Source: CAD feature listing. Evaluate the final solid. Frame: model axes, mm. Face numbers are marked on the shaded views. A direction names the side the tool comes from. Round coordinates to 2 decimals unless told otherwise and drop trailing zeros. Loops run counter-clockwise (first coordinate to the right, second up) from the corner with the lowest first, then second, coordinate; pieces in that order, holes last. Notation, with made-up numbers: M 77.5,53.5 L 122.5,53.5 A33 cw 122.5,90.5 Z; hole C 18.25,71.25 d5. An arc over 180 degrees is marked long. Answer as CSV lines item,"result". Start each with the question number.
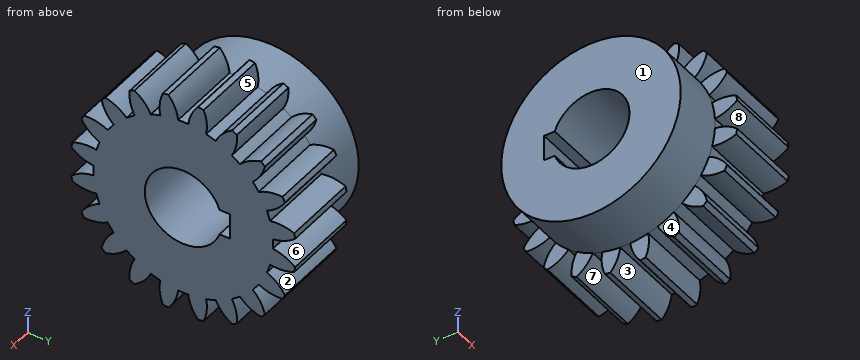
```python
from build123d import *
from build123d.topology import SkipClean

# Parameters (mm, degrees)
BASPROSKE_W      = 30
BASPROSKE_H      = 44
TOOTHCUT_DEPTH   = 70.079664157
TEETHCUTS_COUNT  = 20
TEETHCUTS_ANGLE  = 342
HUBNEARONE_START = 20.0000508
HUBNEAONESKE_R   = 34.999
HUBNEARONE_DEPTH = 20.0000508
BORSKE_R         = 15
BORE_DEPTH       = 50.0000508
KEYSKE_W         = 10
KEYSKE_H         = 18.3
KEYWAY_DEPTH     = 50.0000508


with BuildPart() as part:
    # BasProSke → Base-Revolve (revolve)
    with BuildSketch(Plane(origin=(0, 0, 0), x_dir=(1, 0, 0), z_dir=(0, 1, 0)), mode=Mode.PRIVATE) as base_revolve_sk:
        with Locations((15, 22)):
            Rectangle(BASPROSKE_W, BASPROSKE_H)
    revolve(base_revolve_sk.sketch.rotate(Axis((-10, 0, 0), (1, 0, 0)), 180), axis=Axis((-10, 0, 0), (1, 0, 0)))

    # TooCutSke → ToothCut (cut, through all)
    with BuildSketch(Plane(origin=(0, 0, 0), x_dir=(0, 0, -1), z_dir=(1, 0, 0))):
        with BuildLine():
            ThreePointArc((1.961730392, 34.943978235), (0, 34.999), (-1.961730392, 34.943978235))
            ThreePointArc((-1.961730392, 34.943978235), (-3.235659864, 39.585086827), (-5.832115241, 43.637395396))
            ThreePointArc((-5.832115241, 43.637395396), (0, 44.0254), (5.832115241, 43.637395396))
            ThreePointArc((5.832115241, 43.637395396), (3.235659864, 39.585086827), (1.961730392, 34.943978235))
        make_face()
    toothcut = extrude(amount=TOOTHCUT_DEPTH, mode=Mode.SUBTRACT)

    # TeethCuts: ToothCut ×20 about axis
    teethcuts_axis = Axis((-10, 0, 0), (1, 0, 0))
    for i in range(1, TEETHCUTS_COUNT):
        add(toothcut.rotate(teethcuts_axis, i * TEETHCUTS_ANGLE / (TEETHCUTS_COUNT - 1)), mode=Mode.SUBTRACT)

    # HubNeaOneSke → HubNearOne (add)
    with SkipClean():  # the faces are left unmerged after this step: merging them gives an invalid solid
        with BuildSketch(Plane.ZY.offset(HUBNEARONE_START)):
            Circle(HUBNEAONESKE_R)
        extrude(amount=-HUBNEARONE_DEPTH)

    # BorSke → Bore (cut, symmetric)
    with SkipClean():  # the faces are left unmerged after this step: merging them gives an invalid solid
        with BuildSketch(Plane(origin=(0, 0, 0), x_dir=(0, 0, -1), z_dir=(1, 0, 0))):
            with Locations(Location((0, 0, 0), (0, 0, 180))):
                Circle(BORSKE_R)
        extrude(amount=BORE_DEPTH, both=True, mode=Mode.SUBTRACT)

    # KeySke → Keyway (cut, symmetric)
    with SkipClean():  # the faces are left unmerged after this step: merging them gives an invalid solid
        with BuildSketch(Plane(origin=(0, 0, 0), x_dir=(0, 0, -1), z_dir=(1, 0, 0))):
            with Locations((0, 9.15)):
                Rectangle(KEYSKE_W, KEYSKE_H)
        extrude(amount=KEYWAY_DEPTH, both=True, mode=Mode.SUBTRACT)


solid = part.part
```
1) Section B-B, the plane x = -6. Return loops of the section in (y, z), and give its area (3 significant figures).
2) Access query for the marked faces 4, 5, 6, 7 and 8. Directions: +Z, -Z, +X, -X, +Y, -Y. A direction counts if a zero-diameter tool reaches every point of the face in a straight line with its end or side. Return the directions, or none.
3) Section A-A, the plane y = 0. Return loops of the section in (x, z).
4) Ray query, line 1 along Y through (x, z) = (6.5, -29); line 2 along Z through (x, y) = (-1, 0); line 3 along Y through (x, z) = (-7, 0). Return the intervals inside material, ascending.
5) Mould query, pull axis Z, two halves, no side actions, for the marked faces 1, 2 and 3. Classes: pulls with the +Z half, pulls with the -Z half, needs draft (parallel to the pull), parting line crosses it, or undercut.
6) Contact query for flat-ended pins moving along their axis: pin 1 Ø3.5 at (x, y) = (-2.5, 17) entering from -Z; pin 2 Ø6 at (y, z) = (5.5, 41) entering from -X; pin 3 Ø3 at (x, y) = (-4, -22) entering from -Z. Output: stop coordinate, or through.
7) Section D-D, the plane y = 37. Return loops of the section in (x, z), and give its area (3 significant figures).
8) Section C-C, the plane z = 0. Return loops of the section in (x, y), and give its area (3 significant figures).
Findings below:
1,outline,"C 0,0 d70; hole M 14.14,-5 L 18.3,-5 L 18.3,5 L 14.14,5 A15 ccw long Z"
1,area,"3,110 mm²"
2,face 4,"-Z, -X, -Y"
2,face 5,"+X, -X"
2,face 6,"+X, -X, +Y"
2,face 7,"-Z, +X, -X"
2,face 8,"+X, -X, -Y"
3,outline,"M -20,-35 L 30,-35 L 30,-15 L -20,-15 Z; M -20,15 L 30,15 L 30,35 L -20,35 Z"
4,line 1,"-31.5 to -24.2, -19.59 to 19.59, 24.2 to 31.5"
4,line 2,"-35 to -15, 15 to 35"
4,line 3,"-35 to -15, 18.3 to 35"
5,face 1,"needs draft"
5,face 2,"undercut"
5,face 3,"pulls with the -Z half"
6,pin 1,"z = -31.5"
6,pin 2,"x = 0"
6,pin 3,"z = -28.37"
7,outline,"M 0,-21 L 30,-21 L 30,-15.64 L 0,-15.64 Z; M 0,-9.24 L 30,-9.24 L 30,-2.34 L 0,-2.34 Z; M 0,2.34 L 30,2.34 L 30,9.24 L 0,9.24 Z; M 0,15.64 L 30,15.64 L 30,21 L 0,21 Z"
7,area,"736 mm²"
8,outline,"M -20,-35 L 30,-35 L 30,-15 L -20,-15 Z; M -20,18.3 L 30,18.3 L 30,35 L -20,35 Z"
8,area,"1,830 mm²"
